The drawing under review shows one solid part. Ordinate dimensions are in mm from its lowest x, y, z. Round coordinates to 2 decimals unless told otherwise and drop trailing zeros. Write each loop counter-clockwise with the first axis right and the second up, starting at its lowest first coordinate (ties: lowest second). Pieces come first, ordered by that corner, then holes.
Item 1: Clearance check with flat-ended pins moving along their axes: pin 1 Ø8 at (x, z) = (6.5, 7) entering from +Y; pin 2 Ø0.7 at (y, z) = (1.5, 8.5) entering from -X. State where each tip first meets the part, or that it passes through.
Item 2: Add section A-A (y = 1.55). Give the boundary of the cut face in (x, z).
Item 3: To check wall thickness, follow L1, parallel to Z at x = 2.5, y = 0.2; L2, parallel to X at y = 0.35, z = 10.5; L3, parallel to X at y = 1.9, z = 5.5. State the ranges of each line that lie inside material, in increasing order.
Item 4: Add section B-B (x = 3.5). Give the boundary of the cut face in (y, z), plus the area to 3 significant figures.
Item 5: Add section C-C (z = 10.5). Give the boundary of the cut face in (x, y).
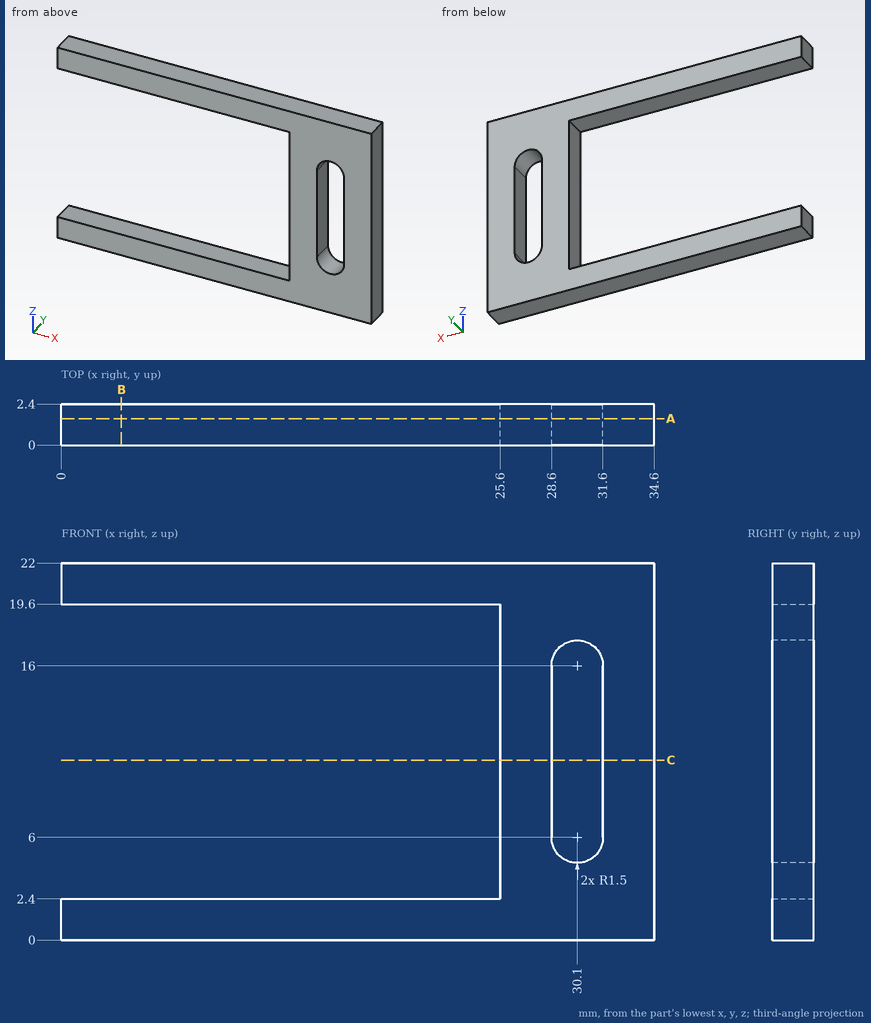
Numbers:
1. pin 1: passes through
1. pin 2: stops at x = 25.6
2. outline: (0, 0) - (34.6, 0) - (34.6, 22) - (0, 22) - (0, 19.6) - (25.6, 19.6) - (25.6, 2.4) - (0, 2.4) - close; hole (28.6, 6) arc R1.5 ccw to (31.6, 6) - (31.6, 16) arc R1.5 ccw to (28.6, 16) - close
3. L1: z = 0 to 2.4, 19.6 to 22
3. L2: x = 25.6 to 28.6, 31.6 to 34.6
3. L3: x = 25.6 to 28.69, 31.51 to 34.6
4. outline: (0, 0) - (2.4, 0) - (2.4, 2.4) - (0, 2.4) - close; (0, 19.6) - (2.4, 19.6) - (2.4, 22) - (0, 22) - close
4. area: 11.5 mm2
5. outline: (25.6, 0) - (28.6, 0) - (28.6, 2.4) - (25.6, 2.4) - close; (31.6, 0) - (34.6, 0) - (34.6, 2.4) - (31.6, 2.4) - close
